```python
from build123d import *

# Parameters (mm, degrees)
SKETCH1_W           = 8.6
SKETCH1_H           = 27.000000000000004
BOSS_EXTRUDE1_DEPTH = 31.5
SKETCH2_W           = 27
SKETCH2_H           = 3
BOSS_EXTRUDE2_DEPTH = 40.5
BOSS_EXTRUDE3_DEPTH = 40.5
BOSS_EXTRUDE4_DEPTH = 31.5
CUT_EXTRUDE6_DEPTH  = 67.48165160403282
SKETCH5_R           = 2.200000000000013
SKETCH5_R_2         = 2.200000000000042
SKETCH5_R_3         = 2.2000000000000135
SKETCH5_R_4         = 2.2000000000000384
CUT_EXTRUDE1_DEPTH  = 5
CUT_EXTRUDE2_DEPTH  = 10
SKETCH8_R           = 5.050000000000001
CUT_EXTRUDE3_DEPTH  = 63.016610678107845
SKETCH9_R           = 1.7500000000000042
CUT_EXTRUDE4_DEPTH  = 8.6
SKETCH10_R          = 3.7500000000000013
CUT_EXTRUDE5_DEPTH  = 6.6
BOSS_EXTRUDE5_START = 2
BOSS_EXTRUDE5_DEPTH = 2
FILLET1_R           = 3
FILLET2_R           = 3
FILLET3_R           = 1
FILLET4_R           = 0.25
FILLET5_R           = 1.5


with BuildPart() as part:
    # Sketch1 → Boss-Extrude1 (new body)
    with BuildSketch(Plane(origin=(0, 0, 0), x_dir=(1, 0, 0), z_dir=(0, 1, 0))):
        Rectangle(SKETCH1_W, SKETCH1_H)
    extrude(amount=BOSS_EXTRUDE1_DEPTH)

    # Sketch2 → Boss-Extrude2 (add)
    with BuildSketch(Plane(origin=(4.3, 0, 0), x_dir=(0, 0, -1), z_dir=(1, 0, 0))):
        with Locations((-1.78e-15, 1.5)):
            Rectangle(SKETCH2_W, SKETCH2_H)
    extrude(amount=BOSS_EXTRUDE2_DEPTH)

    # Sketch3 → Boss-Extrude3 (add)
    with BuildSketch(Plane(origin=(4.3, 0, 0), x_dir=(0, 0, -1), z_dir=(1, 0, 0))):
        Polygon((10.499999999999998, 31.5), (10.500000000000002, 2.9999999999999996), (13.499999999999998, 3), (13.499999999999998, 31.5), align=None)
    extrude(amount=BOSS_EXTRUDE3_DEPTH)

    # Sketch4 → Boss-Extrude4 (add)
    with BuildSketch(Plane(origin=(0, 31.5, 0), x_dir=(1, 0, 0), z_dir=(0, 1, 0))):
        Polygon((44.8, 13.499999999999998), (44.8, -13.5), (53.4, -13.5), (53.4, 13.500000000000004), align=None)
    extrude(amount=-BOSS_EXTRUDE4_DEPTH)

    # Sketch12 → Cut-Extrude6 (cut, through all)
    with BuildSketch(Plane.XY.offset(-10.500000000000002)):
        with BuildLine():
            Line((38.43, 8.25), (38.43, 26.249999999999996))
            ThreePointArc((38.43, 26.249999999999996), (35.93, 28.750000000000004), (33.42999999999999, 26.249999999999996))
            Line((33.42999999999999, 26.249999999999996), (33.42999999999999, 8.25))
            ThreePointArc((33.42999999999999, 8.25), (35.93000000000001, 5.750000000000007), (38.43, 8.25))
        make_face()
        with BuildLine():
            Line((27.049999999999997, 8.25), (27.049999999999997, 26.249999999999996))
            ThreePointArc((27.049999999999997, 26.249999999999996), (24.55, 28.75), (22.049999999999994, 26.249999999999996))
            Line((22.049999999999994, 26.249999999999996), (22.049999999999994, 8.25))
            ThreePointArc((22.049999999999994, 8.25), (24.55, 5.7500000000000036), (27.049999999999997, 8.25))
        make_face()
        with BuildLine():
            Line((15.670000000000003, 8.250000000000014), (15.670000000000003, 26.25))
            ThreePointArc((15.670000000000003, 26.25), (13.170000000000002, 28.75000000000001), (10.669999999999998, 26.25))
            Line((10.669999999999998, 26.25), (10.669999999999998, 8.250000000000014))
            ThreePointArc((10.669999999999998, 8.250000000000014), (13.169999999999995, 5.750000000000018), (15.670000000000003, 8.250000000000014))
        make_face()
    extrude(amount=-CUT_EXTRUDE6_DEPTH, mode=Mode.SUBTRACT)

    # Sketch5 → Cut-Extrude1 (cut)
    with BuildSketch(Plane(origin=(0, 31.5, 0), x_dir=(1, 0, 0), z_dir=(0, 1, 0))):
        with Locations(Location((49.099999999999994, 4.95, 0), (0, 0, 270))):
            Circle(SKETCH5_R)
        with Locations(Location((49.099999999999994, -4.949999999999998, 0), (0, 0, 270))):
            Circle(SKETCH5_R_2)
        with Locations(Location((0, 4.949999999999999, 0), (0, 0, 270))):
            Circle(SKETCH5_R_3)
        with Locations(Location((0, -4.949999999999999, 0), (0, 0, 270))):
            Circle(SKETCH5_R_4)
    extrude(amount=-CUT_EXTRUDE1_DEPTH, mode=Mode.SUBTRACT)

    # Sketch6 → Cut-Extrude2 (cut)
    with BuildSketch(Plane.ZY.offset(-44.8)):
        Polygon((13.5, 26.500000000000004), (13.500000000000014, 5), (-9, 4.999999999999998), (-9, 26.5), align=None)
    extrude(amount=-CUT_EXTRUDE2_DEPTH, mode=Mode.SUBTRACT)

    # Sketch8 → Cut-Extrude3 (cut, through all)
    with BuildSketch(Plane(origin=(0, 3, 0), x_dir=(1, 0, 0), z_dir=(0, 1, 0))):
        with Locations(Location((35.8, -1.75e-15, 0), (0, 0, 270))):
            Circle(SKETCH8_R)
    extrude(amount=-CUT_EXTRUDE3_DEPTH, mode=Mode.SUBTRACT)

    # Sketch9 → Cut-Extrude4 (cut)
    with BuildSketch(Plane.ZY.offset(4.3)):
        with Locations((0, 23.5)):
            Circle(SKETCH9_R)
    extrude(amount=-CUT_EXTRUDE4_DEPTH, mode=Mode.SUBTRACT)

    # Sketch10 → Cut-Extrude5 (cut)
    with BuildSketch(Plane(origin=(4.3, 0, 0), x_dir=(0, 0, -1), z_dir=(1, 0, 0))):
        with Locations((0, 23.5)):
            Circle(SKETCH10_R)
    extrude(amount=-CUT_EXTRUDE5_DEPTH, mode=Mode.SUBTRACT)

    # Sketch11 → Boss-Extrude5 (add)
    with BuildSketch(Plane.ZY.offset(4.3).offset(BOSS_EXTRUDE5_START)):
        with BuildLine():
            Line((-13.5, 21.85), (-13.5, 25.15))
            Line((-13.5, 25.15), (-0.5830951894845463, 25.15))
            ThreePointArc((-0.5830951894845463, 25.15), (-1.750000000000004, 23.5), (-0.5830951894845463, 21.85))
            Line((-0.5830951894845463, 21.85), (-13.5, 21.85))
        make_face()
    extrude(amount=-BOSS_EXTRUDE5_DEPTH)

    # Fillet1
    fillet1_edges = [part.edges().sort_by_distance(p)[0] for p in [
        (44.8, 29, 13.5),
        (53.4, 29, 13.5),
        (53.4, 15.75, -13.500000000000004),
        (53.4, 2.5, 13.5),
        (44.8, 4, 13.5),
        (4.3, 17.25, 13.5),
    ]]
    fillet(fillet1_edges, radius=FILLET1_R)

    # Fillet2
    fillet2_edges = [part.edges().sort_by_distance(p)[0] for p in [
        (-4.3, 10.925, -13.5),
        (-4.3, 15.75, 13.5),
        (-4.3, 28.325, -13.5),
    ]]
    fillet(fillet2_edges, radius=FILLET2_R)

    # Fillet3
    fillet3_edges = [part.edges().sort_by_distance(p)[0] for p in [
        (49.099999999999994, 26.5, -9.000000000000002),
        (49.099999999999994, 4.999999999999998, -9.000000000000002),
    ]]
    fillet(fillet3_edges, radius=FILLET3_R)

    # Fillet4
    fillet4_edges = [part.edges().sort_by_distance(p)[0] for p in [
        (-5.3, 25.15, -0.5830951894845464),
        (-5.3, 21.85, -0.5830951894845464),
    ]]
    fillet(fillet4_edges, radius=FILLET4_R)

    # Fillet5
    fillet5_edges = [part.edges().sort_by_distance(p)[0] for p in [
        (-6.3, 23.5, -13.5),
    ]]
    fillet(fillet5_edges, radius=FILLET5_R)


solid = part.part
```
Model file for the job. Use its own axes, mm. A direction names the side the tool comes from. Give positions to 0.01 mm unless a question says otherwise; leave off trailing zeros. Loops run counter-clockwise (first coordinate to the right, second up) from the corner with the lowest first, then second, coordinate; pieces in that order, holes last. Notation, with made-up numbers: M -32,-36 L 4,-36 A15 cw 4,-19 Z; hole C 17.25,30 d2. An arc over 180 degrees is marked long. Use one line per item in the form item = value.
Item 1: Slice it at B-B on z = 9.25. List the corners of the cut face in (x, y).
Filled in:
outline = M -4.3,0 L 53.4,0 L 53.4,5 L 44.8,5 L 44.8,3 L 4.3,3 L 4.3,31.5 L -4.3,31.5 Z; M 44.8,26.5 L 53.4,26.5 L 53.4,31.5 L 44.8,31.5 Z
Item 2: Two-plate mould, pull along Z, no slides. Class faces 1 (the cylindrical face through (52.54, 15.53, -12.6)), 2 (the flat face through (4.3, 17, 0)), 3 (the flat face through (29, 17, -10.5)), 4 (the cylindrical face through (1.05, 19.84, 0.81)): released by +Z, released by -Z, zero draft, split by the parting line, or undercut.
Filled in:
face_1 = released by -Z
face_2 = zero draft
face_3 = released by +Z
face_4 = undercut
Item 3: Drill centre lines: L1, parallel to Z at x = 49.1, y = 28.75; L2, parallel to X at y = 29.95, z = 4.95; L3, parallel to X at y = 1.6, z = 0. Where is each one in solid material? Low to high.
Filled in:
L1 = -13.5 to -7.15, -2.75 to 2.75, 7.15 to 13.5
L2 = -4.3 to -2.2, 2.2 to 4.3, 44.8 to 46.9, 51.3 to 53.4
L3 = -4.3 to 30.75, 40.85 to 53.4
Item 4: Which spindle directions (+Z, -Z, +X, -X, +Y, -Y) get a long thin tool onto all of the face, cutting with end or side? Do faces 5 (the cylindrical face through (0.66, 29.04, 7.05)), 6 (the flat face through (22.05, 17, -12)), 7 (the flat face through (24, 3, 2)), 8 (the cylindrical face through (-3.44, 28.37, -12.6)), 9 (the cylindrical face through (-3.44, 15.97, 12.6)). Say none if no direction does.
Filled in:
face_5 = +Y
face_6 = +Z, -Z
face_7 = +Z, +Y
face_8 = -Z, -X, +Y
face_9 = +Z, -X, +Y, -Y
Item 5: Slice it at A-A on z = 0. List the corners of the cut face in (x, y).
Filled in:
outline = M -4.3,0 L 30.75,0 L 30.75,3 L 4.3,3 L 4.3,19.75 L -2.3,19.75 L -2.3,21.75 L -4.3,21.75 Z; M -4.3,25.25 L -2.3,25.25 L -2.3,27.25 L 4.3,27.25 L 4.3,31.5 L -4.3,31.5 Z; M 40.85,0 L 53.4,0 L 53.4,5 L 44.8,5 L 44.8,3 L 40.85,3 Z; M 44.8,26.5 L 53.4,26.5 L 53.4,31.5 L 44.8,31.5 Z
Item 6: Slice it at C-C on x = 13.17. List the corners of the cut face in (y, z), and give its area (3 significant figures).
Filled in:
outline = M 0,-13.5 L 5.75,-13.5 L 5.75,-10.5 L 3,-10.5 L 3,13.5 L 0,13.5 Z; M 28.75,-13.5 L 31.5,-13.5 L 31.5,-10.5 L 28.75,-10.5 Z
area = 97.5 mm^2
Item 7: Slice it at D-D on y = 23.5. Give the number of separate pieces and of enclosed holes in the cut face, and give its area (3 significant figures).
Filled in:
separate_pieces = 5
enclosed_holes = 0
area = 308 mm^2
Item 8: Flat gauge pins, fed straight in: pin 1 Ø3.5 at (y, z) = (17.5, -11.5) entering from -X; pin 2 Ø5 at (x, z) = (49.1, 4.95) entering from -Y; pin 3 Ø1 at (x, y) = (40, 22.5) entering from +Z; pin 4 Ø7 at (x, z) = (32, 7) entering from +Y. Where does each tip first touch, or does it go through?
Filled in:
pin_1 = -4.3
pin_2 = 0
pin_3 = -10.5
pin_4 = 3
